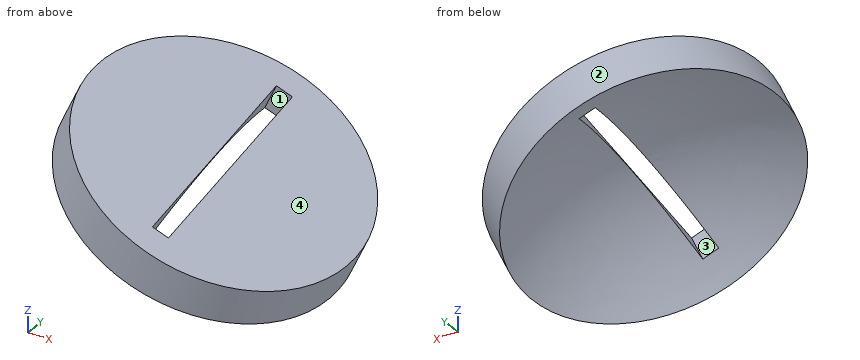
from build123d import *

# Parameters (mm, degrees)
BOX_W               = 3
BOX_H               = 18
BOX_DEPTH           = 40
BOX_PLACEMENT_ANGLE = 20
CUT_ROLL_ANGLE      = -73.158244
CUT_PITCH_ANGLE     = 21.416057
CUT_PLACEMENT_ANGLE = 28.591024


with BuildPart() as slot:
    # Box → Box (new body)
    with BuildSketch(Plane.XY):
        with Locations((1.5, 9)):
            Rectangle(BOX_W, BOX_H)
    extrude(amount=BOX_DEPTH)


with BuildPart() as slot_1:
    # Box placement: moved
    add(slot.part.moved(Location((-8.5, -6, -18))).rotate(Axis((-8.5, -6, -18), (0, 1, 0)), BOX_PLACEMENT_ANGLE))


with BuildPart() as obj1:
    # Sketch → Revolve (revolve)
    with BuildSketch(Plane.XY):
        with BuildLine():
            Line((-25, 0), (0, 0))
            Line((0, 0), (0, 0.410997))
            add(Edge.make_bspline(
                [(0, 0.410997), (-12.5, 0.410997), (-25, 8)],
                knots=[0, 0, 0, 25, 25, 25], degree=2))
            Line((-25, 8), (-25, 0))
        make_face()
    revolve(axis=Axis((0, 0, 0), (0, 1, 0)))

    # Cut: cut slot
    add(slot_1.part, mode=Mode.SUBTRACT)


with BuildPart() as obj1_1:
    # Cut roll: moved
    add(obj1.part.rotate(Axis((0, 0, 0), (1, 0, 0)), CUT_ROLL_ANGLE))


with BuildPart() as obj1_2:
    # Cut pitch: moved
    add(obj1_1.part.rotate(Axis((0, 0, 0), (0, 1, 0)), CUT_PITCH_ANGLE))


with BuildPart() as obj1_3:
    # Cut placement: moved
    add(obj1_2.part.moved(Location((0, 0, 89))).rotate(Axis((0, 0, 89), (0, 0, 1)), CUT_PLACEMENT_ANGLE))


solid = obj1_3.part
Model file for the job. Use its own axes, mm. Face numbers are marked on the shaded views. Coordinates: 2 decimals unless noted, no trailing zeros. Return JSON: item names as keys, results as strings. Group by question number.
Item 1: Flat gauge pins, fed straight in: P1, Ø1.5, axis at x = -1.5, z = 89.5, coming from the +Y side; P2, Ø4, axis at x = -15, y = 16, coming from the -Z side; P3, Ø2, axis at x = 8.5, y = 10, coming from the +Z side; P4, Ø10, axis at x = 14, z = 90, coming from the -Y side. Where does each tip first touch, or does it go through?
Item 2: Wall check: line 1 along Z through (x, y) = (-5.5, 15); line 2 along Z through (x, y) = (15, 16); line 3 along X through (y, z) = (14, 99.25). Give the ranges that are in metal, low to high. Write a range as [from, to].
Item 3: Pull direction X, two halves, no side cores. Call the marked faces 1, 2, 3 and 4: pulls with the +X half, pulls with the -X half, needs draft (parallel to the pull), parting line crosses it, or undercut.
Values found:
{
 "1": {"P1": "stops at y = 25.14", "P2": "stops at z = 90.79", "P3": "stops at z = 86.24", "P4": "passes through"},
 "2": {"line 1": "z = [89.43, 93.22]", "line 2": "z = [75.02, 83.07]", "line 3": "x = [-18, -17.76]"},
 "3": {"face 1": "undercut", "face 2": "parting line crosses it", "face 3": "undercut", "face 4": "pulls with the +X half"}
}
